For this review, use the dimensioned drawing (mm, ordinates from the lowest corner) and the shaded views. Coordinates: 2 decimals unless noted, no trailing zeros. Loops run counter-clockwise (first coordinate to the right, second up) from the corner with the lowest first, then second, coordinate; pieces in that order, holes last. Notation, with made-up numbers: M -14,-14 L 15,-14 A18 cw 15,2 Z; hole C 15.25,16 d11. An arc over 180 degrees is marked long. One line per item, written item: value.
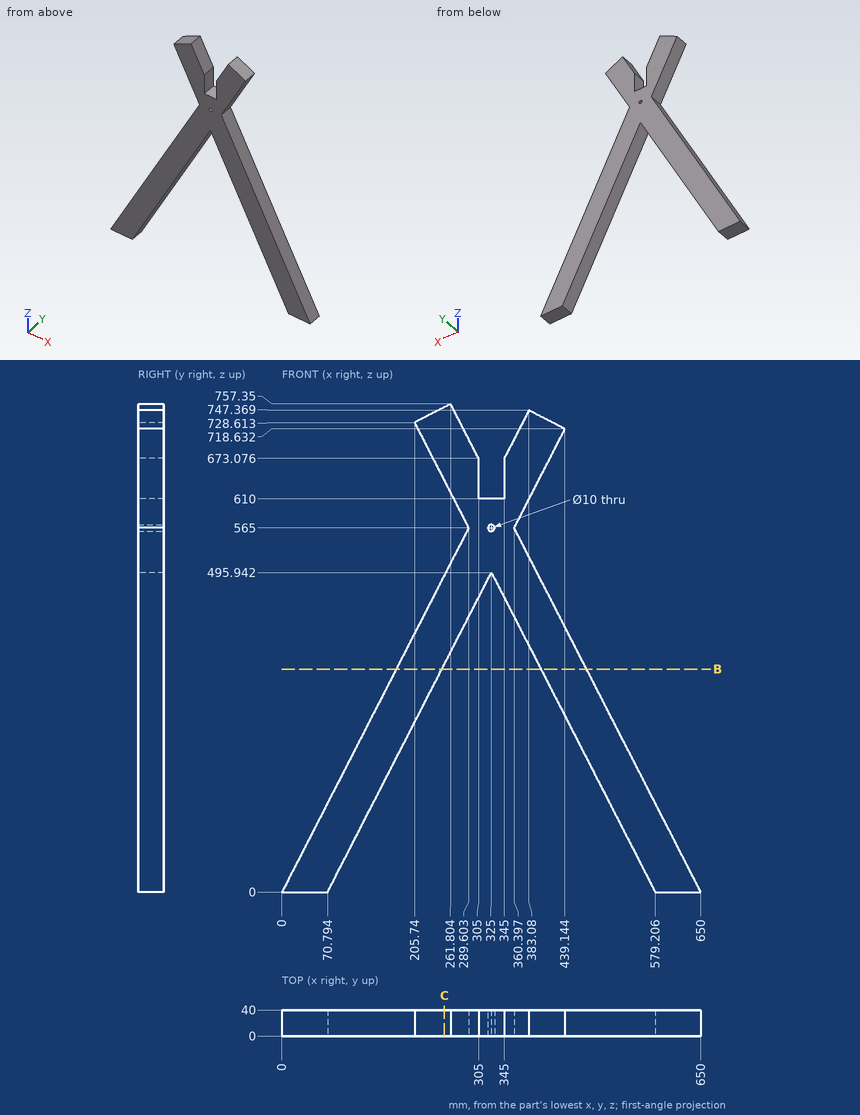
(1) We need section C-C on x = 252. State the section outline as (y, z) points (1 decimal).
Reply:
outline: M 0,353.5 L 40,353.5 L 40,491.6 L 0,491.6 Z; M 0,638.4 L 40,638.4 L 40,752.3 L 0,752.3 Z
(2) We need section B-B on z = 346. State the section outline as (x, y) points, then the cut area to 3 significant figures.
Reply:
outline: M 177.35,0 L 248.14,0 L 248.14,40 L 177.35,40 Z; M 401.86,0 L 472.65,0 L 472.65,40 L 401.86,40 Z
area: 5,660 mm2
(3) Insertion check: pin 1 (20 mm diameter, centred on y = 12.5, z = 636.5, fed in from -X); pin 2 (12 mm diameter, centred on y = 25, z = 643, fed in from +X); pin 3 (8 mm diameter, centred on x = 540.5, y = 17, fed in from +Z) (1 decimal); pin 4 (8 mm diameter, centred on x = 325, z = 565, fed in from +Y). Each pin has a flat end and moves straight along its axis. Give the tip position at first contact, or say it passes through.
Reply:
pin 1: stops at x = 247.83
pin 2: stops at x = 403.45
pin 3: stops at z = 221.4
pin 4: passes through
(4) To check wall thickness, follow line 1 along X through (y, z) = (18, 565); line 2 along X through (y, z) = (19.5, 443.5) (1 decimal); line 3 along Z through (x, y) = (327, 33) (1 decimal). State the ranges of each line that lie inside material, in increasing order. Write a range as [from, to].
Reply:
line 1: x = [289.6, 320], [330, 360.4]
line 2: x = [227.3, 298.1], [351.9, 422.7]
line 3: z = [492, 560.4], [569.6, 610]
